Input: part model. Units: mm. Frame: model coordinates. A direction names the side the tool comes from. Give positions to 0.01 mm unless a question says otherwise; leave off trailing zeros. Write each loop counter-clockwise with the first axis right and the second up, starting at its lowest first coordinate (ties: lowest second). Pieces come first, ordered by that corner, then holes. Notation, with made-up numbers: (1, 13) - (46, 13) arc R21 ccw to (46, 48) - close; hole circle Ø3 at (74.5, 46.25). An arc over 180 degrees is marked (long way). Use a Markdown table: item, result. Add a question column.
1. Section query B-B, the plane x = -1.6. Count the separate pieces of the cut face and the enclosed holes in it, plus the area to 3 significant figures.
2. Section query D-D, the plane y = -0.25. Return loops of the section in (x, z), plus the area to 3 significant figures.
3. Mould query, pull axis Z, two halves, no side actions, for faces 1 (the flat face through (0, -1, 6)), 2 (the cylindrical face through (-0.986, -3.142, 18.692)), 3 (the flat face through (-1.15, 1, -1)). Classes: released by +Z, released by -Z, zero draft, split by the parting line, or undercut.
4. Section query C-C, the plane z = 0. Return loops of the section in (x, y), plus the area to 3 significant figures.
5. Section query A-A, the plane y = -2.25. Return loops of the section in (x, z).
6. Material intervals for probe 1 along Z at (x, y) = (-0.75, 0); probe 2 along Y at (x, z) = (-1.8, -0.5); probe 3 along Y at (x, z) = (-0.65, 0), sorted ascending.
7. Set-up query: faces 4 (the cylindrical face through (-0.99, 4.72, 18.35)), 5 (the cylindrical face through (-0.6, -3, 0.1)). Return all of +Z, -Z, +X, -X, +Y, -Y with unobstructed straight access to the full face (end or side cutting, diameter ignored); none if empty.
Autodesk Inventor part; units mm, degrees
ref_plane "YZ Plane" through (0, 0, 0) normal (1, 0, 0) x (0, 1, 0)
ref_plane "XZ Plane" through (0, 0, 0) normal (0, 1, 0) x (-1, 0, 0)
ref_plane "XY Plane" through (0, 0, 0) normal (0, 0, 1) x (1, 0, 0)
sketch "スケッチ1" plane through (0, 0, 0) normal (1, 0, 0) x (0, 1, 0)
  circle A0 centre (0, 0) radius 3
  circle A1 centre (0, 0) radius 4.5 construction
  circle A2 centre (4.5, 0) radius 0.8
  circle A3 centre (2.25, 3.8971) radius 0.8
  circle A4 centre (-2.25, 3.8971) radius 0.8
  circle A5 centre (-4.5, 0) radius 0.8
  circle A6 centre (-2.25, -3.8971) radius 0.8
  circle A7 centre (2.25, -3.8971) radius 0.8
  line L0 (-25.1126, 0) -> (14.9601, 0)
  line L1 (6.2329, 11) -> (-10, 11)
  line L2 (-10, 11) -> (-7.8852, -1.3502)
  circle A8 centre (0, 0) radius 1.25
  line L3 (0, 0) -> (-10, 0) construction
  line L4 (-10, 0) -> (-10, 11) construction
  arc A9 (-7.8852, -1.3502) -> (7.8852, 1.3502) centre (0, 0) ccw
  line L5 (6.2329, 11) -> (7.8852, 1.3502)
  line L6 (-13.5106, 12.8383) -> (-10.0642, 11.2105)
  line L7 (-10.0642, 11.2105) -> (-7.9495, -1.1398)
  arc A10 (-7.9495, -1.1398) -> (7.821, 1.5607) centre (-0.0642, 0.2105) ccw
  line L8 (7.821, 1.5607) -> (5.0943, 17.4845)
  arc A11 (5.0943, 17.4845) -> (3.9772, 18.9553) centre (3.123, 17.1469) ccw
  line L9 (3.9772, 18.9553) -> (-7.9583, 24.593)
  arc A12 (-7.9583, 24.593) -> (-13.5106, 12.8383) centre (-10.7344, 18.7156) ccw
  circle A13 centre (-0.0642, 0.2105) radius 1
  circle A14 centre (3.123, 17.1469) radius 0.8
  circle A15 centre (-10.7344, 18.7156) radius 3
  arc A16 (-8.4779, 12.0893) -> (-3.8416, 17.4955) centre (-10.7344, 18.7156) ccw
  line L10 (-1.8722, 19.1469) -> (3.123, 19.1469)
  arc A17 (5.0943, 17.4845) -> (3.123, 19.1469) centre (3.123, 17.1469) ccw
  line L11 (-9.8045, 9.8585) -> (-10, 11)
  arc A18 (-1.8722, 19.1469) -> (-3.8416, 17.4955) centre (-1.8722, 17.1469) ccw
  arc A19 (-8.4779, 12.0893) -> (-9.8045, 9.8585) centre (-7.8332, 10.1961) ccw
  point P0 (7.5963, 0)
  point P1 (-10.1271, 11.742)
  point P2 (-3.7477, 19.1469)
  point P3 (-9.6645, 11)
  point P4 (6.2047, 11)
  point P5 (3.9772, 18.9553)
  dimension "d1" = 9
  dimension "d0" = 6
  dimension "d2" = 1.6
  dimension "d5" = 360
  dimension "d8" = 2.5
  dimension "d13" = 8
  dimension "d14" = 10
  dimension "d15" = 11
  dimension "d16" = 7
  dimension "d17" = 2
extrude "押し出し1" add sketch "スケッチ1" against normal blind 2 contours L0 A8 A0 | L0 A2 A10 A9 L2 A5 A0 | A0 L0 A8 | A0 L0 A5 L2 A19 L1 L8 A10 A2 | A10 L8 L1 L5 A9 L0 | L0 A9 A10 | L2 L1 A19 | L1 A19 A16 A18 L10 A17 A11 L8
extrude "押し出し2" cut sketch "スケッチ1" against normal blind 1.15 contours L0 A8 A0 | A0 L0 A8
properties part number "MotorMount"
Result sheet:
| question | item | result |
|---|---|---|
| 1 | separate pieces | 1 |
| 1 | enclosed holes | 8 |
| 1 | area | 349 mm² |
| 2 | outline | (-2, -8) - (0, -8) - (0, -2.99) - (-1.15, -2.99) - (-1.15, -1.22) - (-2, -1.22) - close; (-2, 1.22) - (-1.15, 1.22) - (-1.15, 2.99) - (0, 2.99) - (0, 19.15) - (-2, 19.15) - close |
| 2 | area | 45.3 mm² |
| 3 | face 1 | zero draft |
| 3 | face 2 | released by +Z |
| 3 | face 3 | undercut |
| 4 | outline | (-2, -8.12) - (0, -8.12) - (0, -5.3) - (-2, -5.3) - close; (-2, -3.7) - (0, -3.7) - (0, -3) - (-1.15, -3) - (-1.15, -1.25) - (-2, -1.25) - close; (-2, 1.25) - (-1.15, 1.25) - (-1.15, 3) - (0, 3) - (0, 3.7) - (-2, 3.7) - close; (-2, 5.3) - (0, 5.3) - (0, 8) - (-2, 8) - close |
| 4 | area | 16.8 mm² |
| 5 | outline | (-2, -7.68) - (0, -7.68) - (0, -4.7) - (-2, -4.7) - close; (-2, -3.1) - (0, -3.1) - (0, -1.98) - (-1.15, -1.98) - (-1.15, 1.98) - (0, 1.98) - (0, 3.1) - (-2, 3.1) - close; (-2, 4.7) - (0, 4.7) - (0, 19.11) - (-2, 19.11) - close |
| 6 | probe 1 | z = -8 to -3, 3 to 19.15 |
| 6 | probe 2 | y = -8.03 to -5.12, -3.88 to -1.15, 1.15 to 3.88, 5.12 to 7.98 |
| 6 | probe 3 | y = -8.12 to -5.3, -3.7 to -3, 3 to 3.7, 5.3 to 8 |
| 7 | face 4 | +Z, +X, -X, +Y |
| 7 | face 5 | +X |
